For this review, take the finished solid that the model builds, in its own axes (mm). A direction names the side the tool comes from. Give positions to 0.01 mm unless a question says otherwise; leave off trailing zeros. Write each loop counter-clockwise with the first axis right and the second up, starting at its lowest first coordinate (ties: lowest second). Pieces come first, ordered by that corner, then holes.
Q1. We need section D-D (y = -39.25). Write out the cut boundary in (x, z), then the cut area to 3 significant figures.
Q2. We need section A-A (z = -4.75). Write out the cut boundary in (x, y) (3 decimals), then the cut area to 3 significant figures.
Q3. Machinability: for faces 4 (the flat face through (48, -39, -4)), 5 (the flat face through (41, -42.575, -3)), which of the approach directions +Z, -Z, +X, -X, +Y, -Y give a long, thin tool a straight path to every point of the face, cutting with its end or side? Answer none if there is none.
Q4. Mouldability with a two-part tool opening along X and no side actions: class faces 1 (the cylindrical face through (34.03, -39.817, -1.972)), 2 (the flat face through (51.891, -38.641, -7.063)), 3 (the flat face through (40.737, -38.533, -7.584)) as released by +X, released by -X, zero draft, split by the parting line, or undercut.
Q5. We need section C-C (z = -3.5). Write out the cut boundary in (x, y) (3 decimals), then the cut area to 3 significant figures.
Q6. We need section B-B (x = 34.5). Write out the cut boundary in (y, z) (3 decimals).
Q7. For line 1 (Y direction, x = 33.5, z = -3) (3 decimals); line 2 (X direction, y = -39.5, z = -3.75); line 3 (Y direction, x = 32.5, z = -3) (3 decimals), list the stretches that pass through material, from the lowest coordinate up.
Q8. Insertion check: P1, Ø3, axis at x = 48.5, y = -39, coming from the +Z side. The pin has a flat end and moves straight along its axis. Give the tip position at first contact, or say it passes through.
```python
from build123d import *

# Parameters (mm, degrees)
SKETCH014_W     = 23
SKETCH014_H     = 8
PAD005_DEPTH    = 8
SKETCH015_R     = 1.4
POCKET011_DEPTH = 4
POCKET012_DEPTH = 23.001
FILLET002_R     = 3
CHAMFER_SIZE    = 1


with BuildPart() as part:
    # Sketch014 (on ShapeBinder) → Pad005 (new body)
    with BuildSketch(Plane(origin=(0, 0, 0), x_dir=(1, 0, 0), z_dir=(0, 0, -1))):
        with Locations((40.884375, 38.575)):
            Rectangle(SKETCH014_W, SKETCH014_H)
    extrude(amount=PAD005_DEPTH)

    # Sketch015 (on Face5 of Pad005) → Pocket011 (cut)
    with BuildSketch(Plane.XY):
        with Locations((33.384375, -38.575)):
            Circle(SKETCH015_R)
        with Locations((48.384375, -38.575)):
            Circle(SKETCH015_R)
    extrude(amount=-POCKET011_DEPTH, mode=Mode.SUBTRACT)

    # Sketch016 (on Face2 of Pocket011) → Pocket012 (cut, through all)
    with BuildSketch(Plane(origin=(29.384375, 0, 0), x_dir=(0, -1, 0), z_dir=(-1, 0, 0))):
        Polygon((34.575, -8), (42.575, -7.159166), (42.575, -8), align=None)
    extrude(amount=-POCKET012_DEPTH, mode=Mode.SUBTRACT)

    # Fillet002
    fillet002_edges = [part.edges().sort_by_distance(p)[0] for p in [
        (29.384375, -34.575, -4),
        (52.384375, -34.575, -4),
        (52.384375, -42.575, -3.579583),
        (29.384375, -42.575, -3.579583),
    ]]
    fillet(fillet002_edges, radius=FILLET002_R)

    # Chamfer
    chamfer_edges = [part.edges().sort_by_distance(p)[0] for p in [
        (40.884375, -42.575, -7.159166),
    ]]
    chamfer(chamfer_edges, length=CHAMFER_SIZE)


solid = part.part
```
Computed:
1. outline: (29.38, -6.5) - (30.38, -7.51) - (51.38, -7.51) - (52.38, -6.5) - (52.38, 0) - (49.61, 0) - (49.61, -4) - (47.16, -4) - (47.16, 0) - (34.61, 0) - (34.61, -4) - (32.16, -4) - (32.16, 0) - (29.38, 0) - close
1. area: 152 mm2
2. outline: (29.384, -39.575) arc R3 ccw to (32.384, -42.575) - (49.384, -42.575) arc R3 ccw to (52.384, -39.575) - (52.384, -37.575) arc R3 ccw to (49.384, -34.575) - (32.384, -34.575) arc R3 ccw to (29.384, -37.575) - close
2. area: 176 mm2
3. face 4: +Z
3. face 5: +Z, -Z, +X, -X, -Y
4. face 1: undercut
4. face 2: released by +X
4. face 3: zero draft
5. outline: (29.384, -39.575) arc R3 ccw to (32.384, -42.575) - (49.384, -42.575) arc R3 ccw to (52.384, -39.575) - (52.384, -37.575) arc R3 ccw to (49.384, -34.575) - (32.384, -34.575) arc R3 ccw to (29.384, -37.575) - close; hole circle Ø2.8 at (33.384, -38.575); hole circle Ø2.8 at (48.384, -38.575)
5. area: 164 mm2
6. outline: (-42.575, -6.159) - (-41.58, -7.264) - (-35.57, -7.895) - (-34.575, -7) - (-34.575, 0) - (-37.729, 0) - (-37.729, -4) - (-39.421, -4) - (-39.421, 0) - (-42.575, 0) - close
7. line 1: y = -42.575 to -39.97, -37.18 to -34.575
7. line 2: x = 29.38 to 32.33, 34.44 to 47.33, 49.44 to 52.38
7. line 3: y = -42.575 to -39.66, -37.49 to -34.575
8. P1: stops at z = 0
